Source: CAD feature listing. Evaluate the final solid. Frame: model axes, mm. Face numbers are marked on the shaded views. A direction names the side the tool comes from. Round coordinates to 2 decimals unless told otherwise and drop trailing zeros. Order: outer loops, then holes, each group sorted by start corner. A loop starts at its lowest first (then second) coordinate and runs counter-clockwise, first axis right, second up. Notation, with made-up numbers: (-33.75, 24) - (-27.75, 24) arc R24 ccw to (-27.75, 50) - close; hole circle Ø11 at (51, 66). An arc over 180 degrees is marked (long way). Put each result on its own line as item: value. Start each with the question number.
1) Section A-A on x = -59.5. Output: boundary loops of the cut face in (y, z), then the cut area to 3 significant figures.
2) Mould query, pull axis X, two halves, no side actions, for the marked faces 1, 2 and 3. Classes: +X half, -X half, draft (parallel to the pull), parting line (faces both ways), or undercut.
3) Section B-B on y = 26.7. Output: boundary loops of the cut face in (x, z).
4) Section C-C on z = 1.6. Output: boundary loops of the cut face in (x, y).
5) Contact query for a flat-ended pin moving along its axis: P1, Ø1.5, axis at y = 27.5, z = 1, coming from the -X side. Output: stop coordinate, or through.
6) Line query: probe 1 along X at (y, z) = (25.95, 0.5); probe 2 along X at (y, z) = (25.2, 0.45); probe 3 along Y at (x, z) = (-60, 0.95). Output: solid intervals per line, ascending. Write a range as [from, to].
7) Section D-D on x = -80.5. Output: boundary loops of the cut face in (y, z), then the cut area to 3 significant figures.
8) Access query for the marked faces 4 and 5. Directions: +Z, -Z, +X, -X, +Y, -Y. A direction counts if a zero-diameter tool reaches every point of the face in a straight line with its end or side. Return the directions, or none.
```python
from build123d import *

# Parameters (mm, degrees)
SKETCH1_W           = 30
SKETCH1_H           = 6
SKETCH1_R           = 1.5
BOSS_EXTRUDE1_DEPTH = 3
BOSS_EXTRUDE3_DEPTH = 3


with BuildPart() as part:
    # Sketch1 → Boss-Extrude1 (new body)
    with BuildSketch(Plane.XY):
        with Locations((-68.559747397, 26.091138903)):
            Rectangle(SKETCH1_W, SKETCH1_H)
        with Locations((-81.559747397, 26.091138903)):
            Circle(SKETCH1_R, mode=Mode.SUBTRACT)
        with Locations((-55.559747397, 26.091138903)):
            Circle(SKETCH1_R, mode=Mode.SUBTRACT)
        Polygon((-78.559747397, 26.091138903), (-78.559747397, 27.091138903), (-73.559747397, 27.091138903), (-73.559747397, 25.091138903), (-78.559747397, 25.091138903), align=None, mode=Mode.SUBTRACT)
        Polygon((-58.559747397, 26.091138903), (-58.559747397, 25.091138903), (-63.559747397, 25.091138903), (-63.559747397, 27.091138903), (-58.559747397, 27.091138903), align=None, mode=Mode.SUBTRACT)
    extrude(amount=BOSS_EXTRUDE1_DEPTH)

    # Sketch3 → Boss-Extrude3 (add)
    with BuildSketch(Plane.XY.offset(3)):
        with BuildLine():
            Line((-83.559747397, 26.091138903), (-83.559747397, 28.32720688))
            ThreePointArc((-83.559747397, 28.32720688), (-84.559747397, 26.091138903), (-83.559747397, 23.855070925))
            Line((-83.559747397, 23.855070925), (-83.559747397, 26.091138903))
        make_face()
        with BuildLine():
            Line((-53.559747397, 26.091138903), (-53.559747397, 28.32720688))
            ThreePointArc((-53.559747397, 28.32720688), (-52.559747397, 26.091138903), (-53.559747397, 23.855070925))
            Line((-53.559747397, 23.855070925), (-53.559747397, 26.091138903))
        make_face()
    extrude(amount=-BOSS_EXTRUDE3_DEPTH)


solid = part.part
```
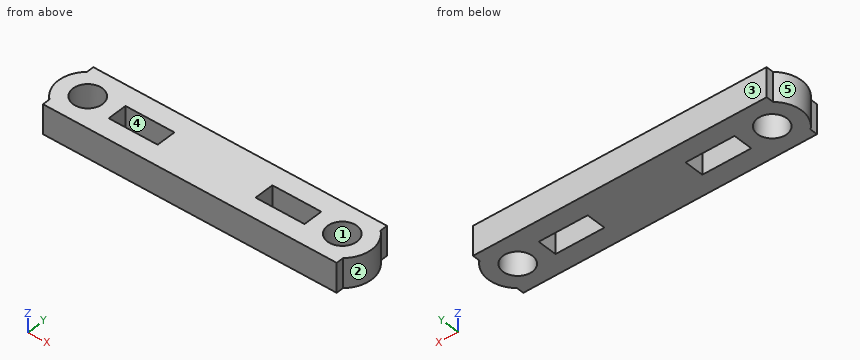
Answer sheet:
1. outline: (23.09, 0) - (25.09, 0) - (25.09, 3) - (23.09, 3) - close; (27.09, 0) - (29.09, 0) - (29.09, 3) - (27.09, 3) - close
1. area: 12.0 mm^2
2. face 1: undercut
2. face 2: +X half
2. face 3: draft
3. outline: (-84.5, 0) - (-82.93, 0) - (-82.93, 3) - (-84.5, 3) - close; (-80.19, 0) - (-78.56, 0) - (-78.56, 3) - (-80.19, 3) - close; (-73.56, 0) - (-63.56, 0) - (-63.56, 3) - (-73.56, 3) - close; (-58.56, 0) - (-56.93, 0) - (-56.93, 3) - (-58.56, 3) - close; (-54.19, 0) - (-52.62, 0) - (-52.62, 3) - (-54.19, 3) - close
4. outline: (-83.56, 23.09) - (-53.56, 23.09) - (-53.56, 23.86) arc R3 ccw to (-53.56, 28.33) - (-53.56, 29.09) - (-83.56, 29.09) - (-83.56, 28.33) arc R3 ccw to (-83.56, 23.86) - close; hole circle Ø3 at (-81.56, 26.09); hole (-78.56, 25.09) - (-73.56, 25.09) - (-73.56, 27.09) - (-78.56, 27.09) - close; hole (-63.56, 25.09) - (-58.56, 25.09) - (-58.56, 27.09) - (-63.56, 27.09) - close; hole circle Ø3 at (-55.56, 26.09)
5. P1: x = -84.49
6. probe 1: [-84.56, -83.05], [-80.07, -78.56], [-73.56, -63.56], [-58.56, -57.05], [-54.07, -52.56]
6. probe 2: [-84.42, -82.77], [-80.35, -78.56], [-73.56, -63.56], [-58.56, -56.77], [-54.35, -52.7]
6. probe 3: [23.09, 25.09], [27.09, 29.09]
7. outline: (23.09, 0) - (25.03, 0) - (25.03, 3) - (23.09, 3) - close; (27.15, 0) - (29.09, 0) - (29.09, 3) - (27.15, 3) - close
7. area: 11.6 mm^2
8. face 4: +Z, -Z
8. face 5: +Z, -Z, -X
